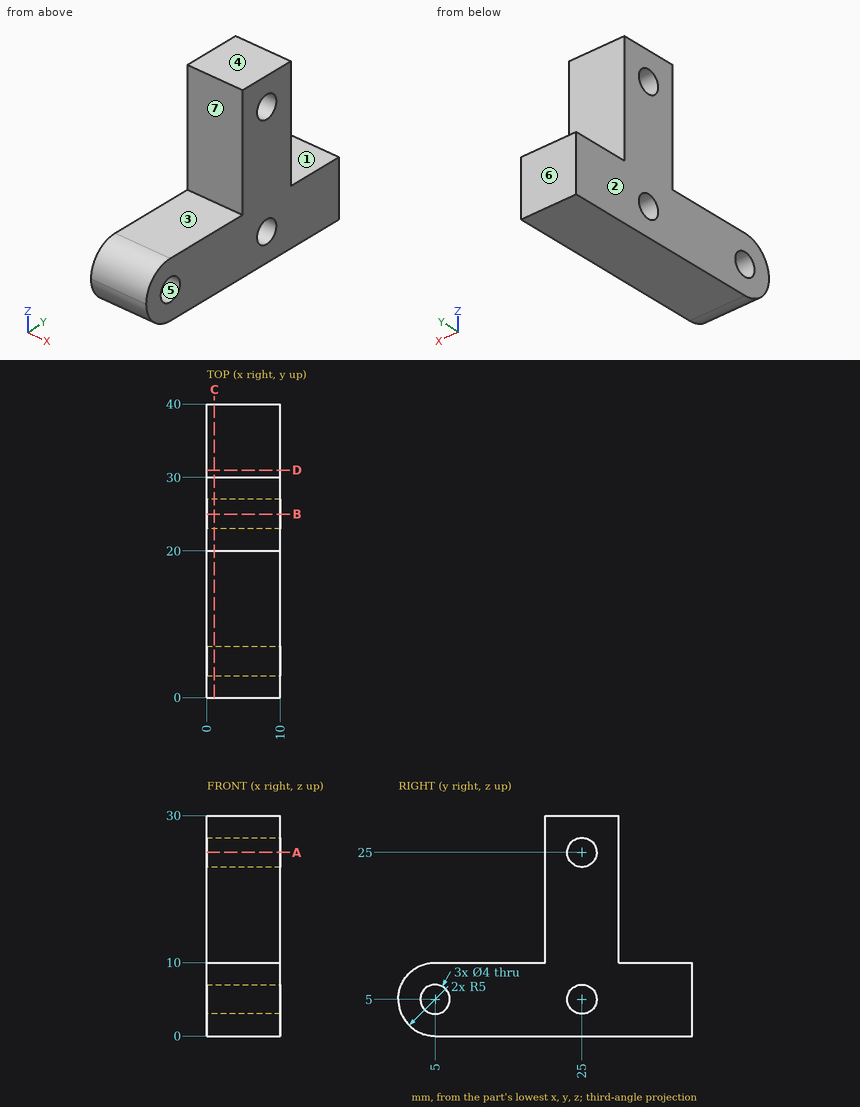
Source: three-view drawing plus pictorial views. Frame: mm from the lowest corner of the part. A direction names the side the tool comes from. Give positions to 0.01 mm unless a question says otherwise; leave off trailing zeros. Loops run counter-clockwise (first coordinate to the right, second up) from the corner with the lowest first, then second, coordinate; pieces in that order, holes last. Notation, with made-up numbers: M 69.5,31.5 L 84.5,31.5 A9 cw 84.5,47.5 Z; hole C 30.5,43.25 d5. An arc over 180 degrees is marked long. Use CSV: the item, a comma, the result in double quotes.
(1) Material intervals for L1, parallel to Y at x = 7.75, z = 5; L2, parallel to Y at x = 8, z = 16; L3, parallel to Z at x = 3, y = 36, sorted ascending. Write a range as [from, to].
Outcome:
L1,"y = [0, 3], [7, 23], [27, 40]"
L2,"y = [20, 30]"
L3,"z = [0, 10]"
(2) Pull-direction query (Y, two-part tool) for the marked faces 4, 5, 6 and 7; classes: pulls with the +Y half, pulls with the -Y half, needs draft (parallel to the pull), parting line crosses it, or undercut.
Outcome:
face 4,"needs draft"
face 5,"undercut"
face 6,"pulls with the +Y half"
face 7,"pulls with the -Y half"
(3) Section B-B, the plane y = 25. Return loops of the section in (x, z), plus the area to 3 significant figures.
Outcome:
outline,"M 0,0 L 10,0 L 10,3 L 0,3 Z; M 0,7 L 10,7 L 10,23 L 0,23 Z; M 0,27 L 10,27 L 10,30 L 0,30 Z"
area,"220 mm²"
(4) Section D-D, the plane y = 31. Return loops of the section in (x, z).
Outcome:
outline,"M 0,0 L 10,0 L 10,10 L 0,10 Z"
(5) Section A-A, the plane z = 25. Return loops of the section in (x, y), plus the area to 3 significant figures.
Outcome:
outline,"M 0,20 L 10,20 L 10,23 L 0,23 Z; M 0,27 L 10,27 L 10,30 L 0,30 Z"
area,"60.0 mm²"
(6) Set-up query: the marked faces 1, 2 and 3. Return all of +Z, -Z, +X, -X, +Y, -Y with unobstructed straight access to the full face (end or side cutting, diameter ignored); none if empty.
Outcome:
face 1,"+Z, +X, -X, +Y"
face 2,"+Z, -Z, -X, +Y, -Y"
face 3,"+Z, +X, -X, -Y"
(7) Pin query (flat end, axial travel): P1, Ø4, axis at x = 4, z = 13, coming from the +Y side; P2, Ø5, axis at y = 25, z = 25, coming from the +X side; P3, Ø2, axis at x = 2.5, y = 7, coming from the +Z side. Return the tip coordinate at first contact, or that it passes through.
Outcome:
P1,"stops at y = 30"
P2,"stops at x = 10"
P3,"stops at z = 10"
(8) Section C-C, the plane x = 1. Count the separate pieces of the cut face and the enclosed holes in it, plus the area to 3 significant figures.
Outcome:
separate pieces,"1"
enclosed holes,"3"
area,"552 mm²"
